```python
from build123d import *

# Parameters (mm, degrees)
CYLINDER014_R             = 4
CYLINDER014_DEPTH         = 10
CYLINDER013_R             = 1.25
CYLINDER013_DEPTH         = 50
PRISM002_DEPTH            = 2.5
BOX004_W                  = 20
BOX004_H                  = 7.25
BOX004_DEPTH              = 10
FILLET004_R               = 3
FILLET005_R               = 3
CYLINDER016_R             = 4
CYLINDER016_DEPTH         = 7.25
CYLINDER015_R             = 9
CYLINDER015_DEPTH         = 7.25
FILLET006_R               = 1
FILLET006_PLACEMENT_ANGLE = 90


with BuildPart() as cylinder013:
    # Cylinder014 → Cylinder014 (new body)
    with BuildSketch(Plane(origin=(0, -16, 22.5), x_dir=(1, 0, 0), z_dir=(0, -1, 0))):
        Circle(CYLINDER014_R)
    extrude(amount=CYLINDER014_DEPTH)


with BuildPart() as fusion004:
    # Cylinder013 → Cylinder013 (new body)
    with BuildSketch(Plane(origin=(0, -16, 22.5), x_dir=(1, 0, 0), z_dir=(0, -1, 0))):
        Circle(CYLINDER013_R)
    extrude(amount=CYLINDER013_DEPTH)

    # Fusion004: union Cylinder013
    add(cylinder013.part)


with BuildPart() as fusion004_1:
    # Fusion004 placement: moved
    add(fusion004.part.moved(Location((0, 57, 0))))


with BuildPart() as fusion005:
    # Prism002 → Prism002 (new body)
    with BuildSketch(Plane(origin=(0, 29, 22.5), x_dir=(1, 0, 0), z_dir=(0, -1, 0))):
        Polygon((3.15, 0), (1.575, 2.72798), (-1.575, 2.72798), (-3.15, 0), (-1.575, -2.72798), (1.575, -2.72798), align=None)
    extrude(amount=PRISM002_DEPTH)

    # Fusion005: union Fusion004
    add(fusion004_1.part)


with BuildPart() as fusion005_1:
    # Fusion005 placement: moved
    add(fusion005.part.moved(Location((0, -26.5, -5))))


with BuildPart() as fillet005:
    # Box004 → Box004 (new body)
    with BuildSketch(Plane(origin=(-10, 0, 12.5), x_dir=(1, 0, 0), z_dir=(0, 0, 1))):
        with Locations((10, 3.625)):
            Rectangle(BOX004_W, BOX004_H)
    extrude(amount=BOX004_DEPTH)

    # Cut012: cut Fusion005
    add(fusion005_1.part, mode=Mode.SUBTRACT)

    # Fillet004
    fillet004_edges = [fillet005.edges().sort_by_distance(p)[0] for p in [
        (10, 3.625, 22.5),
    ]]
    fillet(fillet004_edges, radius=FILLET004_R)

    # Fillet005
    fillet005_edges = [fillet005.edges().sort_by_distance(p)[0] for p in [
        (10, 3.625, 12.5),
        (-10, 3.625, 12.5),
        (-10, 3.625, 22.5),
    ]]
    fillet(fillet005_edges, radius=FILLET005_R)


with BuildPart() as cylinder015:
    # Cylinder016 → Cylinder016 (new body)
    with BuildSketch(Plane(origin=(0, 0, 17.5), x_dir=(1, 0, 0), z_dir=(0, -1, 0))):
        Circle(CYLINDER016_R)
    extrude(amount=CYLINDER016_DEPTH)


with BuildPart() as tornillos_para_metal:
    # Cylinder015 → Cylinder015 (new body)
    with BuildSketch(Plane(origin=(0, 0, 17.5), x_dir=(1, 0, 0), z_dir=(0, -1, 0))):
        Circle(CYLINDER015_R)
    extrude(amount=CYLINDER015_DEPTH)

    # Cut013: cut Cylinder015
    add(cylinder015.part, mode=Mode.SUBTRACT)


with BuildPart() as tornillos_para_metal_1:
    # Cut013 placement: moved
    add(tornillos_para_metal.part.moved(Location((0, 7.25, 0))))

    # Fusion006: union Fillet005
    add(fillet005.part)

    # Fillet006
    fillet006_edges = [tornillos_para_metal_1.edges().sort_by_distance(p)[0] for p in [
        (7.512605, 3.625, 22.455882),
        (7.512605, 3.625, 12.544118),
        (-7.512605, 3.625, 12.544118),
        (-7.512605, 3.625, 22.455882),
    ]]
    fillet(fillet006_edges, radius=FILLET006_R)


with BuildPart() as tornillos_para_metal_2:
    # Fillet006 placement: moved
    add(tornillos_para_metal_1.part.moved(Location((10, 2.5, -2))).rotate(Axis((10, 2.5, -2), (-1, 0, 0)), FILLET006_PLACEMENT_ANGLE))


solid = tornillos_para_metal_2.part
```
Part model, mm, in its own coordinate system. A direction names the side the tool comes from. Coordinates: 2 decimals unless noted, no trailing zeros. Order: outer loops, then holes, each group sorted by start corner. A loop starts at its lowest first (then second) coordinate and runs counter-clockwise, first axis right, second up. Notation, with made-up numbers: (25.25, 28) -> (36.25, 28) arc R30 cw to (36.25, 50) -> close; hole circle Ø4 at (10.5, 50.5). An arc over 180 degrees is marked (long way). Put each result on its own line as item: value. Start each with the question number.
(1) Probe line 1 along X through (y, z) = (20, -6); line 2 along X through (y, z) = (20.5, -5.5); line 3 along Z through (x, y) = (7.25, 22.5). List the from-to ranges inside material, lowest first. Write a range as [from, to].
(2) Pin check, flat tips, straight feed: pin 1 Ø1.5 at (y, z) = (15, -4) entering from +X; pin 2 Ø2 at (x, z) = (8.5, -6.5) entering from -Y. Stop position of each tip, or through.
(3) Band-saw the part on A-A (x = 10). Give the cut face in (y, z), then the cut area to 3 significant figures.
(4) Mould opens along X. For faces 1 (the face through (14.3, 20.1, -9.25)), 2 (the face through (10, 22.728, -3)), 3 (the face through (0, 20, -6)), 4 (the face through (11.4, 20, -4.5)) say: pulls with the +X half, pulls with the -X half, needs draft (parallel to the pull), parting line crosses it, or undercut.
(5) Band-saw the part on D-D (y = 21.5). Give the cut face in (x, z), then the cut area to 3 significant figures.
(6) Band-saw the part on B-B (x = 6.25). Give the cut face in (y, z), then the cut area to 3 significant figures.
(7) Band-saw the part on C-C (y = 23.5). Give the cut face in (x, z).
(8) Which spindle directions (+Z, -Z, +X, -X, +Y, -Y) get a long thin tool onto all of the face, cutting with end or side? Do faces 5 (the face through (20, 20, -6)), 6 (the face through (9, 19, -6.5)), 7 (the face through (10, 17.272, -3)). Say none if no direction does.
Determined:
1. line 1: x = [0, 8.75], [11.25, 20]
1. line 2: x = [0, 8.85], [11.15, 20]
1. line 3: z = [-6.5, -2]
2. pin 1: stops at x = 18.98
2. pin 2: stops at y = 11.01
3. outline: (11, -9.25) -> (16, -9.25) -> (16, -6.5) -> (18.75, -6.5) -> (18.75, -4.5) -> (17.27, -4.5) -> (17.27, -2) -> (11, -2) -> close; (21.25, -6.5) -> (24, -6.5) -> (24, -9.25) -> (29, -9.25) -> (29, -2) -> (22.73, -2) -> (22.73, -4.5) -> (21.25, -4.5) -> close
3. area: 89.9 mm²
4. face 1: needs draft
4. face 2: undercut
4. face 3: pulls with the -X half
4. face 4: undercut
5. outline: (0, -9.25) -> (6.29, -9.25) -> (6.29, -6.5) -> (13.71, -6.5) -> (13.71, -9.25) -> (20, -9.25) -> (20, -2) -> (12.28, -2) -> (12.28, -4.5) -> (7.72, -4.5) -> (7.72, -2) -> (0, -2) -> close
5. area: 113 mm²
6. outline: (11.82, -9.25) -> (18.61, -9.25) -> (18.61, -6.5) -> (21.39, -6.5) -> (21.39, -9.25) -> (28.18, -9.25) -> (28.18, -2) -> (11.82, -2) -> close
6. area: 111 mm²
7. outline: (0.4, -9.25) -> (8.06, -9.25) -> (8.06, -6.5) -> (11.94, -6.5) -> (11.94, -9.25) -> (19.6, -9.25) -> (19.6, -2) -> (0.4, -2) -> close
8. face 5: +Z, -Z, +X, +Y, -Y
8. face 6: -Z
8. face 7: +Z
